Geometry check sheet. Reference: the model listing, model coordinates, mm. Face numbers are marked on the shaded views. A direction names the side the tool comes from. Round coordinates to 2 decimals unless told otherwise and drop trailing zeros. Write each loop counter-clockwise with the first axis right and the second up, starting at its lowest first coordinate (ties: lowest second). Pieces come first, ordered by that corner, then holes. Notation, with made-up numbers: M -2,-9 L 36,-9 A16 ccw 36,12 Z; hole C -3,58.25 d9. An arc over 180 degrees is marked long. Use a Markdown table: item, result.
```python
from build123d import *

# Parameters (mm, degrees)
SKETCH1_R                       = 61.9125
SKETCH1_R_2                     = 35.052
BOSS_EXTRUDE1_DEPTH             = 4.5212
SKETCH3_R                       = 52.3875
BOSS_EXTRUDE2_DEPTH             = 11.43
SKETCH4_R                       = 35.052
CUT_EXTRUDE1_DEPTH              = 89.998629731
SKETCH9_R                       = 36.000000009
CUT_EXTRUDE3_DEPTH              = 8.89
F_5_0MM_DOWEL_HOLE1_D           = 5
F_5_0MM_DOWEL_HOLE1_CSINK_D     = 5.05
F_5_0MM_DOWEL_HOLE1_CSINK_ANGLE = 90
CIRPATTERN1_COUNT               = 60


with BuildPart() as part:
    # Sketch1 → Boss-Extrude1 (new body)
    with BuildSketch(Plane(origin=(0, 0, 0), x_dir=(1, 0, 0), z_dir=(0, 1, 0))):
        with Locations(Location((0, 0, 0), (0, 0, 270))):
            Circle(SKETCH1_R)
        with Locations(Location((0, -12.7, 0), (0, 0, 270))):
            Circle(SKETCH1_R_2, mode=Mode.SUBTRACT)
    extrude(amount=BOSS_EXTRUDE1_DEPTH)

    # Sketch3 → Boss-Extrude2 (add)
    with BuildSketch(Plane(origin=(0, 4.5212, 0), x_dir=(1, 0, 0), z_dir=(0, 1, 0))):
        with Locations(Location((0, 0, 0), (0, 0, 270))):
            Circle(SKETCH3_R)
    extrude(amount=BOSS_EXTRUDE2_DEPTH)

    # Sketch4 → Cut-Extrude1 (cut, through all)
    with BuildSketch(Plane.XZ):
        with Locations(Location((0, 12.7, 0), (0, 0, 270))):
            Circle(SKETCH4_R)
    extrude(amount=-CUT_EXTRUDE1_DEPTH, mode=Mode.SUBTRACT)

    # Sketch9 → Cut-Extrude3 (cut)
    with BuildSketch(Plane(origin=(0, 15.9512, 0), x_dir=(1, 0, 0), z_dir=(0, 1, 0))):
        with Locations(Location((0, -12.7, 0), (0, 0, 270))):
            Circle(SKETCH9_R)
    extrude(amount=-CUT_EXTRUDE3_DEPTH, mode=Mode.SUBTRACT)

    # Ø5.0mm Dowel Hole1 (through all)
    with Locations(Plane(origin=(0, 4.5212, 0), x_dir=(1, 0, 0), z_dir=(0, 1, 0))):
        with Locations((0, 57.15)):
            f_5_0mm_dowel_hole1 = CounterSinkHole(F_5_0MM_DOWEL_HOLE1_D / 2, F_5_0MM_DOWEL_HOLE1_CSINK_D / 2, counter_sink_angle=F_5_0MM_DOWEL_HOLE1_CSINK_ANGLE)

    # CirPattern1: Ø5.0mm Dowel Hole1 ×60 about axis
    cirpattern1_axis = Axis((0, 0, 0), (0, 1, 0))
    for i in range(1, CIRPATTERN1_COUNT):
        add(f_5_0mm_dowel_hole1.rotate(cirpattern1_axis, i * 360 / CIRPATTERN1_COUNT), mode=Mode.SUBTRACT)


solid = part.part
```
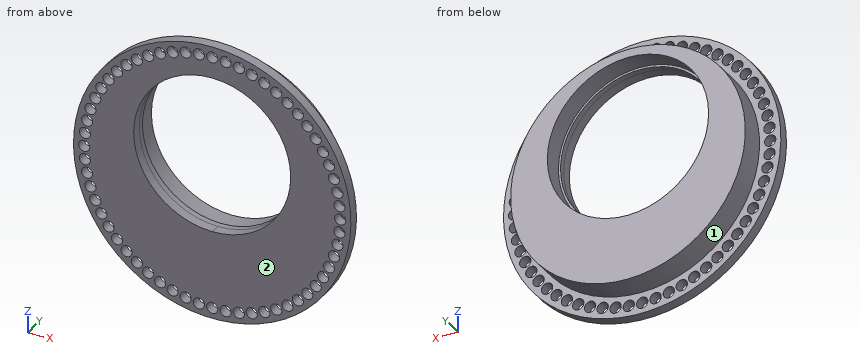
Item 1: Go/stop test with flat-tipped pins: pin 1 (4 mm diameter, centred on x = -17.66, z = 54.35, fed in from +Y); pin 2 (6 mm diameter, centred on x = -49.49, z = -28.58, fed in from +Y); pin 3 (1 mm diameter, centred on y = 2, z = 19, fed in from +X); pin 4 (1 mm diameter, centred on x = 19, y = 6, fed in from -Z). Record where each tip stops, or that it passes through.
Outcome:
| item | result |
|---|---|
| pin 1 | passes through |
| pin 2 | stops at y = 4.52 |
| pin 3 | stops at x = 59.08 |
| pin 4 | stops at z = -49.01 |
Item 2: Cross-section at A-A, the plane y = 9.25. Record the cut outline in (x, z) (1 decimal), and give its area (3 significant figures).
Outcome:
| item | result |
|---|---|
| outline | C 0,0 d104.8; hole C 0,12.7 d72 |
| area | 4,550 mm2 |
Item 3: Access from +Z, -Z, +X, -X, +Y, -Y to the whole of each face (thin tool, end or side, straight path). Record for the marked faces 1 and 2.
Outcome:
| item | result |
|---|---|
| face 1 | +Y |
| face 2 | +Z, -Z, +X, -X, -Y |
Item 4: Material ranges on line 1 along Z through (x, y) = (-18, 1.25); line 2 along Z through (x, y) = (28.5, 8.5); line 3 along Z through (x, y) = (-17.5, 9.5), recorded low to high. Write a range as from..to.
Outcome:
| item | result |
|---|---|
| line 1 | z = -59.24..-56.83, -51.88..-17.38, 42.78..51.88, 56.83..59.24 |
| line 2 | z = -43.96..-9.29, 34.69..43.96 |
| line 3 | z = -49.38..-18.76, 44.16..49.38 |
Item 5: Cross-section at B-B, the plane z = 0. Count the separate pieces of the cut face and the enclosed holes in it, and give its area (3 significant figures).
Outcome:
| item | result |
|---|---|
| separate pieces | 4 |
| enclosed holes | 0 |
| area | 652 mm2 |
